```python
from build123d import *

# Parameters (mm, degrees)
BOSS_EXTRU_1_DEPTH      = 5
ENL_V_MAT_EXTRU_1_DEPTH = 4
ESQUISSE4_R             = 0.9
ENL_V_MAT_EXTRU_2_DEPTH = 10
ESQUISSE3_R             = 0.9
ENL_V_MAT_EXTRU_3_DEPTH = 10


with BuildPart() as part:
    # Esquisse1 → Boss.-Extru.1 (new body)
    with BuildSketch(Plane.XY):
        Polygon((0, 0), (31, 0), (31, -5), (5, -5), (5, -15), (0, -15), align=None)
    extrude(amount=BOSS_EXTRU_1_DEPTH)

    # Esquisse2 → Enlèv. mat.-Extru.1 (cut)
    with BuildSketch(Plane.XY.offset(5)):
        Polygon((1, -15), (5, -15), (5, -5), (31, -5), (31, -1), (1, -1), align=None)
    extrude(amount=-ENL_V_MAT_EXTRU_1_DEPTH, mode=Mode.SUBTRACT)

    # Esquisse4 → Enlèv. mat.-Extru.2 (cut)
    with BuildSketch(Plane.XZ.offset(1)):
        with Locations(Location((26, 3, 0), (0, 0, 270))):
            Circle(ESQUISSE4_R)
        with Locations(Location((6, 3, 0), (0, 0, 270))):
            Circle(ESQUISSE4_R)
    extrude(amount=-ENL_V_MAT_EXTRU_2_DEPTH, mode=Mode.SUBTRACT)

    # Esquisse3 → Enlèv. mat.-Extru.3 (cut)
    with BuildSketch(Plane(origin=(1, 0, 0), x_dir=(0, 0, -1), z_dir=(1, 0, 0))):
        with Locations((-3, -6)):
            Circle(ESQUISSE3_R)
        with Locations((-3, -13)):
            Circle(ESQUISSE3_R)
    extrude(amount=-ENL_V_MAT_EXTRU_3_DEPTH, mode=Mode.SUBTRACT)


solid = part.part
```
Read the model definition and answer for the solid it produces. Units are mm, in the model's axes. A direction names the side the tool comes from. Coordinates: 2 decimals unless noted, no trailing zeros. Write each loop counter-clockwise with the first axis right and the second up, starting at its lowest first coordinate (ties: lowest second). Pieces come first, ordered by that corner, then holes. Notation, with made-up numbers: (89, 16.25) -> (145, 16.25) arc R22 ccw to (145, 46.25) -> close; hole circle Ø10 at (43.5, -17.5). An arc over 180 degrees is marked (long way). Write item = value, one per line.
(1) Given pin 1 Ø2 at (x, y) = (12.5, -7) entering from +Z; pin 2 Ø1.1 at (x, z) = (22.5, 0.5) entering from -Y; pin 3 Ø7 at (x, y) = (13.5, -7.5) entering from +Z; pin 4 Ø2 at (y, z) = (-7.5, 2.5) entering from +X, each flat-ended and moving along its own axis, determine where each tip first touches the part or whether it passes through.
From the geometry:
pin_1 = through
pin_2 = -5
pin_3 = 1
pin_4 = 1
(2) Straight lines are drawn through the part: L1, parallel to Y at x = 0.35, z = 3; L2, parallel to Z at x = 15.5, y = -1.5; L3, parallel to Y at x = 14.5, z = 4.05. For each, find the intervals that lie inside material, in ascending order. Write a range as from..to.
From the geometry:
L1 = -15..-13.9, -12.1..-6.9, -5.1..0
L2 = 0..1
L3 = -1..0
(3) Section D-D on x = 19 is taken. Write down the section's boundary in (y, z), plus the area to 3 significant figures.
From the geometry:
outline = (-5, 0) -> (0, 0) -> (0, 5) -> (-1, 5) -> (-1, 1) -> (-5, 1) -> close
area = 9.00 mm2
(4) Section A-A on y = -13 is taken. Write down the section's boundary in (x, z), plus the area to 3 significant figures.
From the geometry:
outline = (0, 0) -> (5, 0) -> (5, 1) -> (1, 1) -> (1, 2.1) -> (0, 2.1) -> close; (0, 3.9) -> (1, 3.9) -> (1, 5) -> (0, 5) -> close
area = 7.20 mm2
(5) Section B-B on z = 3 is taken. Write down the section's boundary in (x, y), plus the area to 3 significant figures.
From the geometry:
outline = (0, -15) -> (1, -15) -> (1, -13.9) -> (0, -13.9) -> close; (0, -12.1) -> (1, -12.1) -> (1, -6.9) -> (0, -6.9) -> close; (0, -5.1) -> (1, -5.1) -> (1, -1) -> (5.1, -1) -> (5.1, 0) -> (0, 0) -> close; (6.9, -1) -> (25.1, -1) -> (25.1, 0) -> (6.9, 0) -> close; (26.9, -1) -> (31, -1) -> (31, 0) -> (26.9, 0) -> close
area = 37.8 mm2
(6) Section C-C on x = 26 is taken. Write down the section's boundary in (y, z).
From the geometry:
outline = (-5, 0) -> (0, 0) -> (0, 2.1) -> (-1, 2.1) -> (-1, 1) -> (-5, 1) -> close; (-1, 3.9) -> (0, 3.9) -> (0, 5) -> (-1, 5) -> close
(7) For a pull along Y with two mould halves and no side action, classify faces 1 (the face through (0.507, -6.798, 2.585)), 2 (the face through (15, 0, 2)), 3 (the face through (12, -4, 0)) as +Y half, -Y half, draft (parallel to the pull), parting line (faces both ways), or undercut.
From the geometry:
face_1 = undercut
face_2 = +Y half
face_3 = draft
(8) Which of the six approach directions +Z, -Z, +X, -X, +Y, -Y give full straight-line access (tool end or side, diameter ignored) to faces 4 (the face through (5, -9.9, 0.5)), 5 (the face through (6.27, -0.51, 2.14)), 6 (the face through (16, -1, 3))?
From the geometry:
face_4 = +Z, -Z, +X, -Y
face_5 = +Y, -Y
face_6 = +Z, +X, -Y
